```python
from build123d import *

# Parameters (mm, degrees)
F0_W     = 88.9
F0_H     = 12.7
F1_DEPTH = 12.7
F2_W     = 83.82
F2_H     = 7.62
F3_DEPTH = 10.16
F4_T     = -2.54
F5_W     = 12.7
F5_H     = 7.62
F6_DEPTH = 25.4
F7_R     = 3.81
F8_DEPTH = 25.4


with BuildPart() as f1:
    # F0 (on Top) → F1 (new body)
    with BuildSketch(Plane.XY):
        with Locations((3.885043, 20.237593)):
            Rectangle(F0_W, F0_H)
    extrude(amount=F1_DEPTH)

    # F2 (on face) → F3 (join)
    with BuildSketch(Plane.XY.offset(12.7)):
        with Locations((3.885043, 20.237593)):
            Rectangle(F2_W, F2_H)
    extrude(amount=-F3_DEPTH)

    # F4
    f4_openings = [f1.faces().sort_by_distance(p)[0] for p in [
        (3.885043, 20.237593, 12.7),
    ]]
    offset(amount=F4_T, openings=f4_openings)

    # F5 (on face) → F6 (cut)
    with BuildSketch(Plane(origin=(0, 0, 0), x_dir=(1, 0, 0), z_dir=(0, 0, -1))):
        with Locations((41.985043, -20.237593)):
            Rectangle(F5_W, F5_H)
    extrude(amount=-F6_DEPTH, mode=Mode.SUBTRACT)

    # F7 (on face) → F8 (cut)
    with BuildSketch(Plane(origin=(0, 26.587593, 0), x_dir=(-1, 0, 0), z_dir=(0, 1, 0))):
        with Locations((-41.985043, 6.35)):
            Circle(F7_R)
    extrude(amount=-F8_DEPTH, mode=Mode.SUBTRACT)


solid = f1.part
```
Here's how the part is built. I have some questions about the finished solid (model axes, mm). A direction names the side the tool comes from. Coordinates: 2 decimals unless noted, no trailing zeros. Order: outer loops, then holes, each group sorted by start corner. A loop starts at its lowest first (then second) coordinate and runs counter-clockwise, first axis right, second up.
Item 1: I'm going to push flat-ended pins straight in: pin 1 Ø2.5 at (x, y) = (-1.5, 20.5) entering from +Z; pin 2 Ø3 at (y, z) = (19.5, 1.5) entering from +X. Where does each tip first touch, or does it pass through?
Response values:
pin 1: stops at z = 2.54
pin 2: stops at x = 35.64
Item 2: Which directions (+Z, -Z, +X, -X, +Y, -Y) give clear straight access to the entire face, cutting with the end or side of a thin tool? Please do faces 4 (the face through (-2, 20, 2.54)), 5 (the face through (3, 26.588, 6)).
Response values:
face 4: +Z, +X
face 5: +Z, -Z, +X, -X, +Y
Item 3: Thinking about a two-plate mould opening in X: for faces 1 (the face through (35.635, 20, 1)), 2 (the face through (5, 24.048, 8)), 3 (the face through (42.481, 15.175, 10.128)), which applies, pulls with the +X half, pulls with the -X half, needs draft (parallel to the pull), parting line crosses it, or undercut?
Response values:
face 1: pulls with the +X half
face 2: needs draft
face 3: undercut
Item 4: If we section it at A-A, the plane x = 37: List the corners of the cut face in (y, z) for me.
Response values:
outline: (13.89, 0) - (16.43, 0) - (16.43, 12.7) - (13.89, 12.7) - close; (24.05, 0) - (26.59, 0) - (26.59, 12.7) - (24.05, 12.7) - close
Item 5: If we section it at B-B, the plane z = 6.35: List the corners of the cut face in (x, y) for me, then the cut area to 3 significant figures.
Response values:
outline: (-40.56, 13.89) - (38.18, 13.89) - (38.18, 16.43) - (-38.02, 16.43) - (-38.02, 24.05) - (38.18, 24.05) - (38.18, 26.59) - (-40.56, 26.59) - close; (45.8, 13.89) - (48.34, 13.89) - (48.34, 16.43) - (45.8, 16.43) - close; (45.8, 24.05) - (48.34, 24.05) - (48.34, 26.59) - (45.8, 26.59) - close
area: 432 mm2
Item 6: If we section it at D-D, the plane x = -20: List the corners of the cut face in (y, z) for me, then the cut area to 3 significant figures.
Response values:
outline: (13.89, 0) - (26.59, 0) - (26.59, 12.7) - (24.05, 12.7) - (24.05, 2.54) - (16.43, 2.54) - (16.43, 12.7) - (13.89, 12.7) - close
area: 83.9 mm2
Item 7: If we section it at C-C, the plane z = 11.75: List the corners of the cut face in (x, y) for me, then the cut area to 3 significant figures.
Response values:
outline: (-40.56, 13.89) - (48.34, 13.89) - (48.34, 16.43) - (-38.02, 16.43) - (-38.02, 24.05) - (48.34, 24.05) - (48.34, 26.59) - (-40.56, 26.59) - close
area: 471 mm2
Item 8: I need wall thicknesses on probe 1 along Y at (x, z) = (42, 11.25); probe 2 along Z at (x, y) = (24, 18.5); probe 3 along X at (y, z) = (20, 1.25). Which ranges of each line are inside material? Lowest first, please.
Response values:
probe 1: y = 13.89 to 16.43, 24.05 to 26.59
probe 2: z = 0 to 2.54
probe 3: x = -40.56 to 35.64
